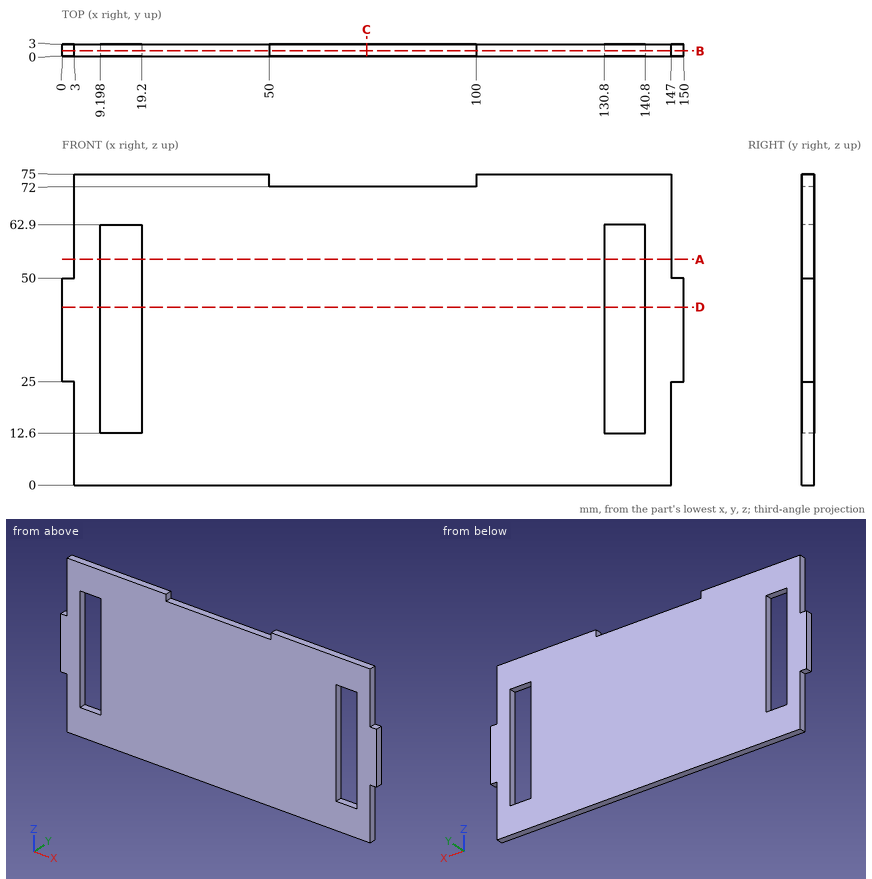
Answer from the drawing. Dimensions are ordinates in mm from the lowest x, y and z of the part. Coordinates: 2 decimals unless noted, no trailing zeros. Order: outer loops, then holes, each group sorted by start corner. A loop starts at its lowest first (then second) coordinate and runs counter-clockwise, first axis right, second up. Notation, with made-up numbers: (62.25, -15.75) - (68.25, -15.75) arc R14 cw to (68.25, 0.25) - close; hole circle Ø5 at (75, -8.5). An arc over 180 degrees is marked (long way). Put each result on its own line as item: value. Start each with the question number.
1) Find section D-D (z = 43). Give the vertices of the cut face in (x, y), plus the area to 3 significant figures.
2) Find the intervals of material crossed by line 1 (X direction, y = 0.75, z = 23.5); line 2 (X direction, y = 1.95, z = 28); line 3 (X direction, y = 2.85, z = 69), in increasing order. Write a range as from..to.
3) Flat-ended cylindrical pins translate along their axes: pin 1 (1.5 mm diameter, centred on y = 1.5, z = 73, fed in from -X); pin 2 (1.5 mm diameter, centred on y = 2, z = 73.5, fed in from +X); pin 3 (0.9 mm diameter, centred on x = 1.5, y = 2, fed in from +Z). Find the tip coordinate at first contact, or state that the pin passes through.
4) Find section C-C (x = 73.5). Give the vertices of the cut face in (y, z).
5) Find section A-A (z = 54.5). Give the vertices of the cut face in (x, y).
6) Find section B-B (y = 1.35). Give the vertices of the cut face in (x, z).
Results list:
1. outline: (0, 0) - (9.2, 0) - (9.2, 3) - (0, 3) - close; (19.2, 0) - (130.8, 0) - (130.8, 3) - (19.2, 3) - close; (140.8, 0) - (150, 0) - (150, 3) - (140.8, 3) - close
1. area: 390 mm^2
2. line 1: x = 3..9.2, 19.2..130.8, 140.8..147
2. line 2: x = 0..9.2, 19.2..130.8, 140.8..150
2. line 3: x = 3..147
3. pin 1: stops at x = 3
3. pin 2: stops at x = 147
3. pin 3: stops at z = 50
4. outline: (0, 0) - (3, 0) - (3, 72) - (0, 72) - close
5. outline: (3, 0) - (9.2, 0) - (9.2, 3) - (3, 3) - close; (19.2, 0) - (130.8, 0) - (130.8, 3) - (19.2, 3) - close; (140.8, 0) - (147, 0) - (147, 3) - (140.8, 3) - close
6. outline: (0, 25) - (3, 25) - (3, 0) - (147, 0) - (147, 25) - (150, 25) - (150, 50) - (147, 50) - (147, 75) - (100, 75) - (100, 72) - (50, 72) - (50, 75) - (3, 75) - (3, 50) - (0, 50) - close; hole (9.2, 12.6) - (19.2, 12.6) - (19.2, 62.9) - (9.2, 62.9) - close; hole (130.8, 12.6) - (140.8, 12.6) - (140.8, 62.9) - (130.8, 62.9) - close
